Geometry: see drawing. Coordinates: mm, zero at the bounding-box minimum. Round coordinates to 2 decimals unless told otherwise and drop trailing zeros. Loops run counter-clockwise (first coordinate to the right, second up) from the corner with the lowest first, then second, coordinate; pieces in that order, holes last. Notation, with made-up numbers: M 26,73 L 35,73 A12 ccw 35,82 Z; hole C -19.5,28 d1. An arc over 180 degrees is marked long. Answer as a JSON object with one key per item and string values.
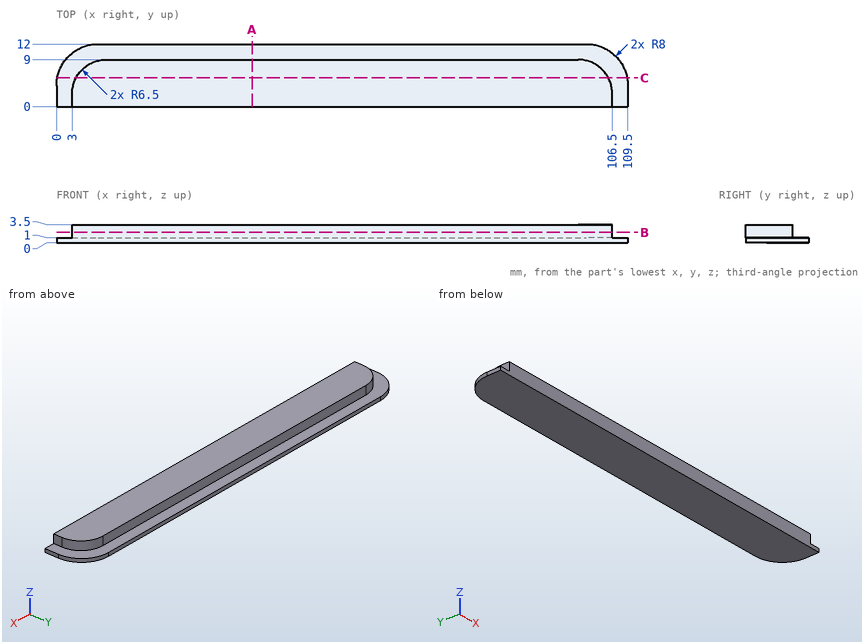
1) Section query C-C (y = 5.5). Return the cut outline in (x, z), and give its area (3 significant figures).
Results:
{"outline": "M 0.14,0 L 109.36,0 L 109.36,1 L 105.77,1 L 105.77,3.5 L 3.73,3.5 L 3.73,1 L 0.14,1 Z", "area": "364 mm2"}
2) Section query A-A (x = 37.5). Return the cut outline in (y, z), and give its area (3 significant figures).
Results:
{"outline": "M 0,0 L 12,0 L 12,1 L 9,1 L 9,3.5 L 0,3.5 Z", "area": "34.5 mm2"}
3) Ray query, line 1 (Y direction, x = 81, z = 3.15); line 2 (X direction, y = 1.75, z = 2.7); line 3 (Z direction, x = 5.5, y = 8.5). Return the intervals inside material, ascending.
Results:
{"line 1": "0 to 9", "line 2": "3 to 106.5", "line 3": "0 to 1"}
4) Pin query (flat end, axial travel): P1, Ø3, axis at x = 76.5, y = 4.5, coming from the -Z side; P2, Ø1.2, axis at y = 1, z = 2, coming from the +X side. Return the tip coordinate at first contact, or that it passes through.
Results:
{"P1": "z = 0", "P2": "x = 106.5"}
5) Section query B-B (z = 2). Return the cut outline in (x, y).
Results:
{"outline": "M 3,0 L 106.5,0 L 106.5,2.5 A6.5 ccw 100,9 L 9.5,9 A6.5 ccw 3,2.5 Z"}
